Check sheet for the modelled part. Datum: model origin and axes. Units: mm. Face numbers are marked on the shaded views. Coordinates: 2 decimals unless noted, no trailing zeros. Loops run counter-clockwise (first coordinate to the right, second up) from the corner with the lowest first, then second, coordinate; pieces in that order, holes last. Notation, with made-up numbers: M 12.5,73.5 L 29.5,73.5 A10 ccw 29.5,78.5 Z; hole C 12,49.25 d7. An arc over 180 degrees is marked long. Write each question's results on one line, items separated by ' | '. Start each with the question number.
from build123d import *

# Parameters (mm, degrees)
SKETCH1_R                 = 14.2875
BOSS_EXTRUDE1_DEPTH       = 19.05
FILLET1_R                 = 5.08
SHELL1_T                  = -1.5875
F_8_CLEARANCE_HOLE1_D     = 4.4958
F_8_CLEARANCE_HOLE1_DEPTH = 6.35
F_8_CLEARANCE_HOLE1_TIP   = 1.350674586


with BuildPart() as part:
    # Sketch1 → Boss-Extrude1 (new body)
    with BuildSketch(Plane(origin=(0, 0, 0), x_dir=(1, 0, 0), z_dir=(0, 1, 0))):
        with Locations(Location((0, 0, 0), (0, 0, 90))):
            Circle(SKETCH1_R)
    extrude(amount=BOSS_EXTRUDE1_DEPTH)

    # Fillet1
    fillet1_edges = [part.edges().sort_by_distance(p)[0] for p in [
        (0, 0, 14.2875),
    ]]
    fillet(fillet1_edges, radius=FILLET1_R)

    # Shell1
    shell1_openings = [part.faces().sort_by_distance(p)[0] for p in [
        (0, 19.05, 0),
    ]]
    offset(amount=SHELL1_T, openings=shell1_openings, kind=Kind.INTERSECTION)

    # #8 Clearance Hole1
    with Locations(Plane(origin=(0, 1.5875, 0), x_dir=(1, 0, 0), z_dir=(0, 1, 0))):
        with Locations((0, 0)):
            Hole(F_8_CLEARANCE_HOLE1_D / 2, depth=F_8_CLEARANCE_HOLE1_DEPTH)
            with Locations((0, 0, -(F_8_CLEARANCE_HOLE1_DEPTH + F_8_CLEARANCE_HOLE1_TIP / 2))):  # 118° drill point
                Cone(0, F_8_CLEARANCE_HOLE1_D / 2, F_8_CLEARANCE_HOLE1_TIP, mode=Mode.SUBTRACT)


solid = part.part
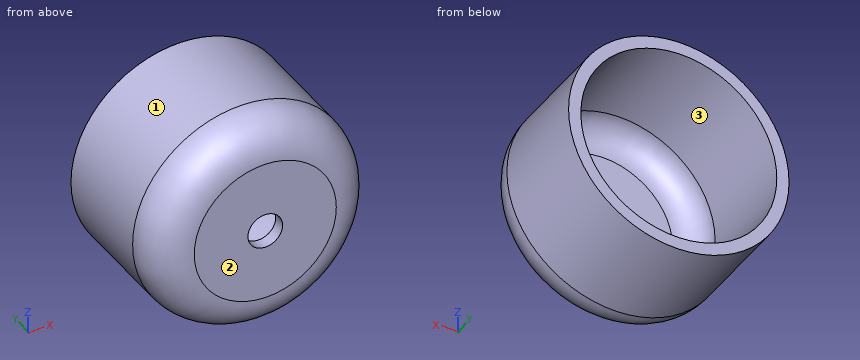
Item 1: Depth check by flat-ended pin: P1, Ø1.5, axis at x = -7.5, z = 8, coming from the -Y side; P2, Ø1, axis at y = 5, z = -0.5, coming from the -X side; P3, Ø4, axis at x = 9, z = -11, coming from the -Y side; P4, Ø9, axis at x = 4.5, z = -2.5, coming from the +Y side. Enter the tip coordinate at first touch or a pass-through.
Item 2: Release check for a two-part mould opening along Z. For the marked faces 1, 2 and 3 record: +Z half, -Z half, draft (parallel to the pull), parting line (faces both ways), or undercut.
Item 3: Section check B-B (y = 6.75). Record the cut outline in (x, z) (1 decimal), plus the area to 3 significant figures.
Item 4: Thickness scan on line 1 (Z direction, x = 0.25, y = 11); line 2 (Y direction, x = -6.25, z = -5.75). Record the ranges inside material, lowest first.
Computed values:
1) P1: stops at y = 0.1 | P2: stops at x = -14.29 | P3: stops at y = 0.98 | P4: stops at y = 1.62
2) face 1: parting line | face 2: draft | face 3: undercut
3) outline: C 0,0 d28.6; hole C 0,0 d25.4 | area: 135 mm²
4) line 1: z = -14.29 to -12.7, 12.7 to 14.29 | line 2: y = 0 to 1.59
